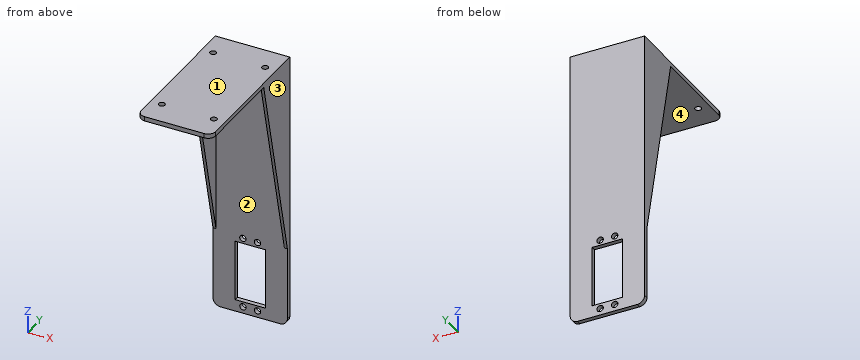
```python
from build123d import *

# Parameters (mm, degrees)
SKETCH_1_W          = 50
SKETCH_1_H          = 187
EXTRUDE_1_DEPTH     = 3
SKETCH_4_R          = 2.15
SKETCH_4_W          = 20.5
SKETCH_4_H          = 41
CUT_EXTRUDE_2_DEPTH = 4
SKETCH_5_W          = 50
SKETCH_5_H          = 3
EXTRUDE_2_DEPTH     = 96
SKETCH_6_R          = 2.1
CUT_EXTRUDE_3_DEPTH = 188
FILLET_1_R          = 5
EXTRUDE_3_DEPTH     = 2
EXTRUDE_4_DEPTH     = 2


with BuildPart() as part:
    # 草图1 → 凸台-拉伸1 (new body)
    with BuildSketch(Plane(origin=(0, 0, 0), x_dir=(1, 0, 0), z_dir=(0, 1, 0))):
        Rectangle(SKETCH_1_W, SKETCH_1_H)
    extrude(amount=EXTRUDE_1_DEPTH)

    # 草图4 → 切除-拉伸2 (cut, through all)
    with BuildSketch(Plane.XZ):
        with Locations((-4.9, -89)):
            Circle(SKETCH_4_R)
        with Locations((4.9, -89)):
            Circle(SKETCH_4_R)
        with Locations((4.9, -41)):
            Circle(SKETCH_4_R)
        with Locations((-4.9, -41)):
            Circle(SKETCH_4_R)
        with Locations((0, -65)):
            Rectangle(SKETCH_4_W, SKETCH_4_H)
    extrude(amount=-CUT_EXTRUDE_2_DEPTH, mode=Mode.SUBTRACT)

    # 草图5 → 凸台-拉伸2 (add)
    with BuildSketch(Plane.XZ):
        with Locations((0, 92)):
            Rectangle(SKETCH_5_W, SKETCH_5_H)
    extrude(amount=EXTRUDE_2_DEPTH)

    # 草图6 → 切除-拉伸3 (cut, through all)
    with BuildSketch(Plane.XY.offset(93.5)):
        with Locations((-17.5, -14)):
            Circle(SKETCH_6_R)
        with Locations((17.5, -14)):
            Circle(SKETCH_6_R)
        with Locations((17.5, -79)):
            Circle(SKETCH_6_R)
        with Locations((-17.5, -79)):
            Circle(SKETCH_6_R)
    extrude(amount=-CUT_EXTRUDE_3_DEPTH, mode=Mode.SUBTRACT)

    # 圆角1
    fillet_1_edges = [part.edges().sort_by_distance(p)[0] for p in [
        (-25, -96, 92),
        (25, -96, 92),
        (-25, 1.5, -93.5),
        (25, 1.5, -93.5),
    ]]
    fillet(fillet_1_edges, radius=FILLET_1_R)

    # 草图7 → 凸台-拉伸3 (add)
    with BuildSketch(Plane(origin=(25, 0, 0), x_dir=(0, 0, -1), z_dir=(1, 0, 0))):
        Polygon((39.5, 0), (-90.5, -30), (-90.5, 0), align=None)
    extrude(amount=-EXTRUDE_3_DEPTH)

    # 草图9 → 凸台-拉伸4 (add)
    with BuildSketch(Plane.ZY.offset(25)):
        Polygon((-39.5, 0), (90.5, -30), (90.5, 0), align=None)
    extrude(amount=-EXTRUDE_4_DEPTH)


solid = part.part
```
The model under review builds one solid part; all positions refer to its coordinate system, in mm. Face numbers are marked on the shaded views. Round coordinates to 2 decimals unless told otherwise and drop trailing zeros. Write each loop counter-clockwise with the first axis right and the second up, starting at its lowest first coordinate (ties: lowest second). Pieces come first, ordered by that corner, then holes.
(1) Mouldability with a two-part tool opening along X and no side actions: class the marked faces 1, 2, 3 and 4 as +X half, -X half, draft (parallel to the pull), parting line (faces both ways), or undercut.
(2) We need section B-B on z = -48. Give the boundary of the cut face in (x, y), and give its area (3 significant figures).
(3) We need section C-C on y = -4. Give the boundary of the cut face in (x, z).
(4) We need section A-A on x = 4.9. Give the boundary of the cut face in (y, z).
(5) We need section D-D on x = 13. Give the boundary of the cut face in (y, z), and give its area (3 significant figures).
(6) Insertion check: pin 1 (5 mm diameter, centred on x = 17.5, y = -79, fed in from -Z); pin 2 (5 mm diameter, centred on x = 13.5, z = 39.5, fed in from -Y); pin 3 (5.5 mm diameter, centred on x = -17.5, y = -79, fed in from +Z). Each pin has a flat end and moves straight along its axis. Give the tip position at first contact, or say it passes through.
(7) Wall thickness on L1, parallel to Z at x = 4.9, y = 0.7; L2, parallel to Y at x = 17.5, z = 91.3; L3, parallel to X at y = -4.5, z = 22: over which ranges is each line inside the solid? List them lowest first.
Findings below:
1. face 1: draft
1. face 2: undercut
1. face 3: +X half
1. face 4: undercut
2. outline: (-25, 0) - (-10.25, 0) - (-10.25, 3) - (-25, 3) - close; (10.25, 0) - (25, 0) - (25, 3) - (10.25, 3) - close
2. area: 88.5 mm2
3. outline: (-25, -22.17) - (-23, -22.17) - (-23, 90.5) - (23, 90.5) - (23, -22.17) - (25, -22.17) - (25, 93.5) - (-25, 93.5) - close
4. outline: (-96, 90.5) - (0, 90.5) - (0, -38.85) - (3, -38.85) - (3, 93.5) - (-96, 93.5) - close; (0, -93.5) - (3, -93.5) - (3, -91.15) - (0, -91.15) - close; (0, -86.85) - (3, -86.85) - (3, -85.5) - (0, -85.5) - close; (0, -44.5) - (3, -44.5) - (3, -43.15) - (0, -43.15) - close
5. outline: (-96, 90.5) - (0, 90.5) - (0, -93.5) - (3, -93.5) - (3, 93.5) - (-96, 93.5) - close
5. area: 849 mm2
6. pin 1: stops at z = 90.5
6. pin 2: stops at y = 0
6. pin 3: stops at z = 93.5
7. L1: z = -93.5 to -91.15, -86.85 to -85.5, -44.5 to -43.15, -38.85 to 93.5
7. L2: y = -96 to -81.1, -76.9 to -16.1, -11.9 to 3
7. L3: x = -25 to -23, 23 to 25
